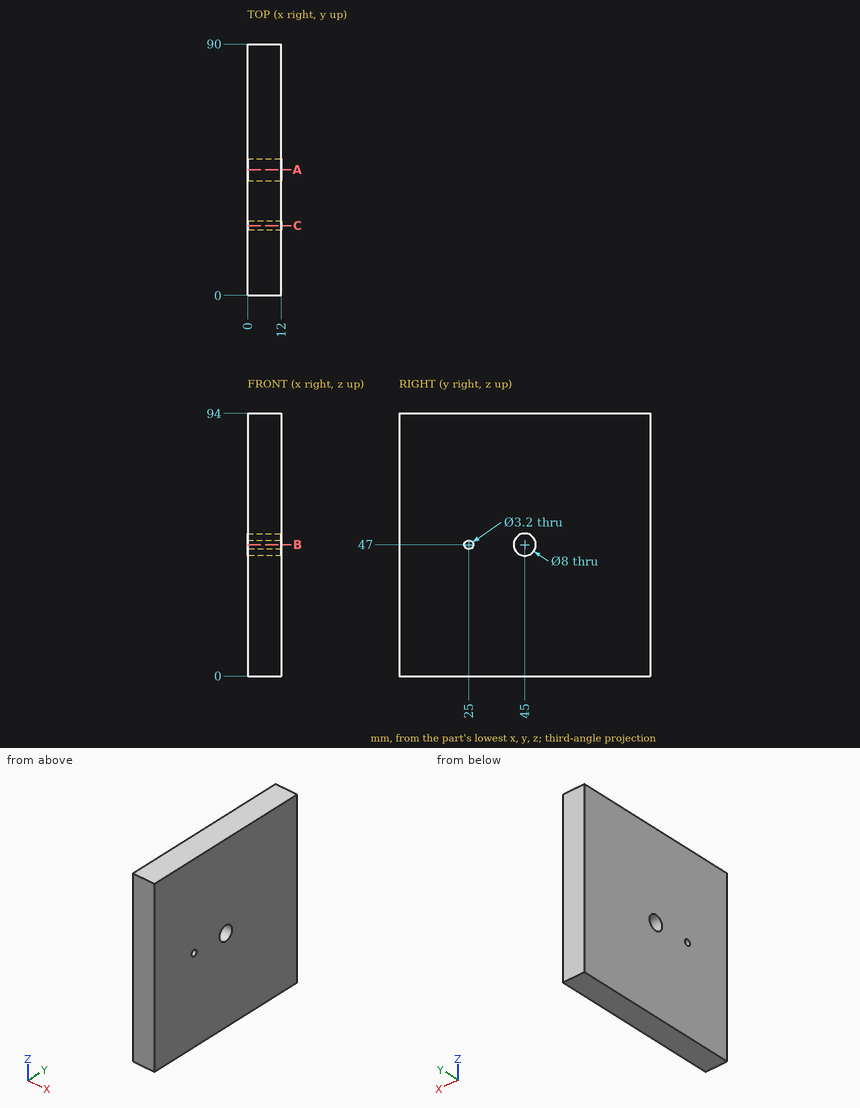
Can you work these out from the drawing? Everything is in mm from the part's minimum corner. Coordinates: 2 decimals unless noted, no trailing zeros. Loops run counter-clockwise (first coordinate to the right, second up) from the corner with the lowest first, then second, coordinate; pieces in that order, holes last. Notation, with made-up numbers: (87, 68.25) - (113, 68.25) arc R21 ccw to (113, 106.25) - close; hole circle Ø10 at (69, 10). An arc over 180 degrees is marked (long way). Answer as CSV lines item,"result".
Q1. If we section it at C-C, the plane y = 25: Write out the boundary of the cut face in (x, z), and give its area (3 significant figures).
Response:
outline,"(0, 0) - (12, 0) - (12, 45.4) - (0, 45.4) - close; (0, 48.6) - (12, 48.6) - (12, 94) - (0, 94) - close"
area,"1,090 mm2"
Q2. If we section it at B-B, the plane z = 47: Write out the boundary of the cut face in (x, y).
Response:
outline,"(0, 0) - (12, 0) - (12, 23.4) - (0, 23.4) - close; (0, 26.6) - (12, 26.6) - (12, 41) - (0, 41) - close; (0, 49) - (12, 49) - (12, 90) - (0, 90) - close"
Q3. If we section it at A-A, the plane y = 45: Write out the boundary of the cut face in (x, z).
Response:
outline,"(0, 0) - (12, 0) - (12, 43) - (0, 43) - close; (0, 51) - (12, 51) - (12, 94) - (0, 94) - close"
Q4. If I drill on L1, parallel to Y at x = 6, z = 47; L2, parallel to Z at x = 6.25, y = 26; L3, parallel to Y at x = 5.5, z = 44, over which ranges is the centre line in solid material (lowest first)? Write a range as [from, to].
Response:
L1,"[0, 23.4], [26.6, 41], [49, 90]"
L2,"[0, 45.75], [48.25, 94]"
L3,"[0, 42.35], [47.65, 90]"
